The listing builds one solid part. Answer for the finished solid, in the listing's coordinates (mm). A direction names the side the tool comes from. Give positions to 0.01 mm unless a question says otherwise; leave off trailing zeros. Write each loop counter-clockwise with the first axis right and the second up, starting at its lowest first coordinate (ties: lowest second). Pieces come first, ordered by that corner, then holes. Notation, with made-up numbers: (27.5, 28) - (80.5, 28) arc R20 cw to (80.5, 67) - close; hole circle Ø1 at (44, -12). An arc over 180 degrees is marked (long way). Return JSON: item names as keys, results as strings.
from build123d import *

# Parameters (mm, degrees)
SKETCH1_W           = 19
SKETCH1_H           = 20
SKETCH1_W_2         = 2
SKETCH1_H_2         = 5
BOSS_EXTRUDE1_DEPTH = 2
SKETCH2_W           = 5
SKETCH2_H           = 15
CUT_EXTRUDE1_DEPTH  = 10
CUT_EXTRUDE3_DEPTH  = 10


with BuildPart() as part:
    # Sketch1 → Boss-Extrude1 (new body)
    with BuildSketch(Plane(origin=(0, 0, 0), x_dir=(1, 0, 0), z_dir=(0, 1, 0))):
        with Locations((5.5, 0)):
            Rectangle(SKETCH1_W, SKETCH1_H)
        with Locations((-1, 5)):
            Rectangle(SKETCH1_W_2, SKETCH1_H_2, mode=Mode.SUBTRACT)
        with Locations((-1, -5)):
            Rectangle(SKETCH1_W_2, SKETCH1_H_2, mode=Mode.SUBTRACT)
    extrude(amount=BOSS_EXTRUDE1_DEPTH)

    # Sketch2 → Cut-Extrude1 (cut)
    with BuildSketch(Plane(origin=(0, 2, 0), x_dir=(1, 0, 0), z_dir=(0, 1, 0))):
        with Locations((2.5, 0)):
            Rectangle(SKETCH2_W, SKETCH2_H)
    extrude(amount=-CUT_EXTRUDE1_DEPTH, mode=Mode.SUBTRACT)

    # Sketch3 → Cut-Extrude3 (cut)
    with BuildSketch(Plane(origin=(0, 2, 0), x_dir=(1, 0, 0), z_dir=(0, 1, 0))):
        Polygon((-4, 10), (-2, 10), (-2, 3.892371719), (1.539535597, 3.892371719), (1.539535597, -3.189870508), (-2, -3.189870508), (-2, -10), (-4, -10), align=None)
    extrude(amount=-CUT_EXTRUDE3_DEPTH, mode=Mode.SUBTRACT)


solid = part.part
Item 1: A cutting plane is placed at C-C on z = 1. Determine the outline of the cut face in (x, y), then the cut area to 3 significant figures.
Answer below:
{"outline": "(5, 0) - (15, 0) - (15, 2) - (5, 2) - close", "area": "20.0 mm²"}
Item 2: A cutting plane is placed at A-A on x = 0.75. Determine the outline of the cut face in (y, z).
Answer below:
{"outline": "(0, -10) - (2, -10) - (2, -7.5) - (0, -7.5) - close; (0, 7.5) - (2, 7.5) - (2, 10) - (0, 10) - close"}
Item 3: For faces 5 (the face through (8, 0, 0)), 6 (the face through (1, 1, 7.5)), determine the directions among +Z, -Z, +X, -X, +Y, -Y from which every point of the face is accessible in a straight line to the end or side of a thin tool.
Answer below:
{"face 5": "+Z, -Z, +X, -X, -Y", "face 6": "-X, +Y, -Y"}
Item 4: The mould has two halves that part along Z. Classify faces 1 (the face through (6, 1, 10)), 2 (the face through (5, 1, 0)), 3 (the face through (6, 1, -10)), 4 (the face through (-2, 1, -9)): +Z half, -Z half, draft (parallel to the pull), parting line (faces both ways), or undercut.
Answer below:
{"face 1": "+Z half", "face 2": "undercut", "face 3": "-Z half", "face 4": "draft"}
Item 5: Consider L1, parallel to Z at x = 2.75, y = 0.2; L2, parallel to X at y = 1.1, z = 0.75. Determine where each line is inside the solid, lowest interval first.
Answer below:
{"L1": "z = -10 to -7.5, 7.5 to 10", "L2": "x = 5 to 15"}
Item 6: A cutting plane is placed at B-B on y = 1.4. Determine the outline of the cut face in (x, z), then the cut area to 3 significant figures.
Answer below:
{"outline": "(-2, -10) - (15, -10) - (15, 10) - (-2, 10) - (-2, 7.5) - (5, 7.5) - (5, -7.5) - (-2, -7.5) - close", "area": "235 mm²"}
Item 7: A flat-ended cylindrical pin translates along its axis: P1, Ø1, axis at y = 1, z = -0.5, coming from the -X side. Find the tip coordinate at first contact, or state that the pin passes through.
Answer below:
{"P1": "stops at x = 5"}
